from build123d import *

# Parameters (mm, degrees)
SKETCH1_W            = 40
SKETCH1_H            = 30
BOSS_EXTRUDE1_DEPTH  = 2
CHAMFER1_SIZE        = 2
N_CUT_EXTRUDE1_DEPTH = 51.039984013
N_CUT_EXTRUDE2_DEPTH = 51.039984013
D_DIAMETER_HOLE1_D   = 4.5


with BuildPart() as part:
    # Sketch1 → Boss-Extrude1 (new body)
    with BuildSketch(Plane.XY):
        with Locations((20, 15)):
            Rectangle(SKETCH1_W, SKETCH1_H)
    extrude(amount=BOSS_EXTRUDE1_DEPTH)

    # Chamfer1
    chamfer1_edges = [part.edges().sort_by_distance(p)[0] for p in [
        (0, 30, 1),
        (40, 30, 1),
        (40, 0, 1),
        (0, 0, 1),
    ]]
    chamfer(chamfer1_edges, length=CHAMFER1_SIZE)

    # Sketch2 → N Cut-Extrude1 (cut, through all)
    with BuildSketch(Plane.XY.offset(2)):
        with BuildLine():
            Line((5, 7.75), (15, 7.75))
            ThreePointArc((15, 7.75), (16.75, 6), (15, 4.25))
            Line((15, 4.25), (5, 4.25))
            ThreePointArc((5, 4.25), (3.25, 6), (5, 7.75))
        make_face()
    extrude(amount=-N_CUT_EXTRUDE1_DEPTH, mode=Mode.SUBTRACT)

    # Sketch3 → N Cut-Extrude2 (cut, through all)
    with BuildSketch(Plane.XY.offset(2)):
        with BuildLine():
            Line((5, 25.75), (15, 25.75))
            ThreePointArc((15, 25.75), (16.75, 24), (15, 22.25))
            Line((15, 22.25), (5, 22.25))
            ThreePointArc((5, 22.25), (3.25, 24), (5, 25.75))
        make_face()
    extrude(amount=-N_CUT_EXTRUDE2_DEPTH, mode=Mode.SUBTRACT)

    # D Diameter Hole1 (through all)
    with Locations(Plane.XY.offset(2)):
        with Locations((35, 15)):
            Hole(D_DIAMETER_HOLE1_D / 2)


solid = part.part
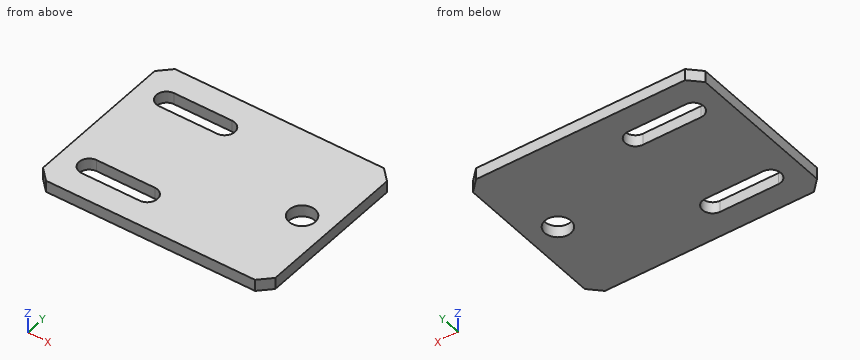
Part model, mm, in its own coordinate system. Give positions to 0.01 mm unless a question says otherwise; leave off trailing zeros. Loops run counter-clockwise (first coordinate to the right, second up) from the corner with the lowest first, then second, coordinate; pieces in that order, holes last. Notation, with made-up numbers: (-7.75, 15) -> (25.25, 15) arc R21 ccw to (25.25, 54) -> close; hole circle Ø11 at (13, -30). An arc over 180 degrees is marked (long way). Write each question's results on one line, items separated by ' | '. Start each with the question number.
Q1. Band-saw the part on D-D on z = 1.1. List the corners of the cut face in (x, y).
Q2. Band-saw the part on B-B on y = 15. List the corners of the cut face in (x, z).
Q3. Band-saw the part on C-C on x = 35. List the corners of the cut face in (y, z), plus the area to 3 significant figures.
Q4. Band-saw the part on A-A on x = 13. List the corners of the cut face in (y, z).
Q5. Wall check: L1, parallel to Y at x = 35, z = 1.6; L2, parallel to Y at x = 4, z = 0.9; L3, parallel to X at y = 23.5, z = 0.15. Give the ranges that are in metal, low to high.
Results are:
1) outline: (0, 2) -> (2, 0) -> (38, 0) -> (40, 2) -> (40, 28) -> (38, 30) -> (2, 30) -> (0, 28) -> close; hole (5, 4.25) -> (15, 4.25) arc R1.75 ccw to (15, 7.75) -> (5, 7.75) arc R1.75 ccw to start; hole (5, 22.25) -> (15, 22.25) arc R1.75 ccw to (15, 25.75) -> (5, 25.75) arc R1.75 ccw to start; hole circle Ø4.5 at (35, 15)
2) outline: (0, 0) -> (32.75, 0) -> (32.75, 2) -> (0, 2) -> close; (37.25, 0) -> (40, 0) -> (40, 2) -> (37.25, 2) -> close
3) outline: (0, 0) -> (12.75, 0) -> (12.75, 2) -> (0, 2) -> close; (17.25, 0) -> (30, 0) -> (30, 2) -> (17.25, 2) -> close | area: 51.0 mm²
4) outline: (0, 0) -> (4.25, 0) -> (4.25, 2) -> (0, 2) -> close; (7.75, 0) -> (22.25, 0) -> (22.25, 2) -> (7.75, 2) -> close; (25.75, 0) -> (30, 0) -> (30, 2) -> (25.75, 2) -> close
5) L1: y = 0 to 12.75, 17.25 to 30 | L2: y = 0 to 4.56, 7.44 to 22.56, 25.44 to 30 | L3: x = 0 to 3.32, 16.68 to 40
